Work out the finished part from the listing and answer in its coordinate system (mm). Coordinates: 2 decimals unless noted, no trailing zeros. Order: outer loops, then holes, each group sorted by start corner. A loop starts at its lowest first (then second) coordinate and runs counter-clockwise, first axis right, second up. Notation, with made-up numbers: M 48,29.25 L 107,29.25 A24 ccw 107,57.25 Z; hole C 38,60.25 d7. An arc over 180 degrees is marked long. Use a Markdown table: item, result.
from build123d import *

# Parameters (mm, degrees)
SKETCH1_R               = 5
BOSS_EXTRUDE1_DEPTH     = 80
BOSS_EXTRUDE2_START     = 80
SKETCH2_W               = 44.999999916
SKETCH2_H               = 12.5
BOSS_EXTRUDE2_DEPTH     = 12.5
CUT_EXTRUDE1_DEPTH      = 96.402109506
CUT_EXTRUDE1_DEPTH_BACK = 96.402109506
SKETCH3_W               = 0.3
SKETCH3_H               = 10


with BuildPart() as part:
    # Sketch1 → Boss-Extrude1 (new body)
    with BuildSketch(Plane(origin=(0, 0, 0), x_dir=(1, 0, 0), z_dir=(0, 1, 0))):
        with Locations(Location((0, 0, 0), (0, 0, 270))):
            Circle(SKETCH1_R)
    extrude(amount=BOSS_EXTRUDE1_DEPTH)

    # Sketch2 → Boss-Extrude2 (add)
    with BuildSketch(Plane(origin=(0, 0, 0), x_dir=(1, 0, 0), z_dir=(0, 1, 0)).offset(BOSS_EXTRUDE2_START)):
        Rectangle(SKETCH2_W, SKETCH2_H)
    extrude(amount=BOSS_EXTRUDE2_DEPTH)

    # Sketch3 → Cut-Extrude1 (cut, two sides: drawn at the far end of the back side and taken through both)
    with BuildSketch(Plane(origin=(0, 0, 0), x_dir=(0, 0, -1), z_dir=(1, 0, 0)).offset(-CUT_EXTRUDE1_DEPTH_BACK)):
        with Locations((0, 87.5)):
            Rectangle(SKETCH3_W, SKETCH3_H)
    extrude(amount=CUT_EXTRUDE1_DEPTH + CUT_EXTRUDE1_DEPTH_BACK, mode=Mode.SUBTRACT)


solid = part.part
(1) Straight lines are drawn through the part: L1, parallel to Y at x = 12.5, z = -0.75; L2, parallel to X at y = 21, z = 0.25; L3, parallel to Z at x = -2.5, y = 73. For each, find the intervals that lie inside material, in ascending order.
Conclusion:
| item | result |
|---|---|
| L1 | 80 to 92.5 |
| L2 | -4.99 to 4.99 |
| L3 | -4.33 to 4.33 |
(2) Determine the mould class of faces 1 (the flat face through (0, 87, -0.15)), 2 (the cylindrical face through (-4.88, 39.44, -1.08)), 3 (the flat face through (0, 92.5, 3)), 4 (the flat face through (0, 87, 0.15)) for opening direction Z: pulls with the +Z half, pulls with the -Z half, needs draft (parallel to the pull), parting line crosses it, or undercut.
Conclusion:
| item | result |
|---|---|
| face 1 | undercut |
| face 2 | parting line crosses it |
| face 3 | needs draft |
| face 4 | undercut |
(3) A cutting plane is placed at C-C (x = 0). Determine the outline of the cut face in (y, z).
Conclusion:
| item | result |
|---|---|
| outline | M 0,-5 L 80,-5 L 80,-6.25 L 92.5,-6.25 L 92.5,-0.15 L 82.5,-0.15 L 82.5,0.15 L 92.5,0.15 L 92.5,6.25 L 80,6.25 L 80,5 L 0,5 Z |
(4) Given P1, Ø6, axis at y = 19, z = 2.5, coming from the -X side; P2, Ø4, axis at y = 30, z = 2, coming from the +X side; P3, Ø1.5, axis at y = 73.5, z = -3, coming from the +X side, each flat-ended and moving along its own axis, determine where each tip first touches the part or whether it passes through.
Conclusion:
| item | result |
|---|---|
| P1 | x = -5 |
| P2 | x = 5 |
| P3 | x = 4.47 |
(5) A cutting plane is placed at D-D (y = 45). Determine the outline of the cut face in (x, z), then the cut area to 3 significant figures.
Conclusion:
| item | result |
|---|---|
| outline | C 0,0 d10 |
| area | 78.5 mm2 |
(6) A cutting plane is placed at B-B (z = -2.25). Determine the outline of the cut face in (x, y).
Conclusion:
| item | result |
|---|---|
| outline | M -22.5,80 L -4.47,80 L -4.47,0 L 4.47,0 L 4.47,80 L 22.5,80 L 22.5,92.5 L -22.5,92.5 Z |
(7) A cutting plane is placed at A-A (y = 87). Determine the outline of the cut face in (x, z), then the cut area to 3 significant figures.
Conclusion:
| item | result |
|---|---|
| outline | M -22.5,-6.25 L 22.5,-6.25 L 22.5,-0.15 L -22.5,-0.15 Z; M -22.5,0.15 L 22.5,0.15 L 22.5,6.25 L -22.5,6.25 Z |
| area | 549 mm2 |
